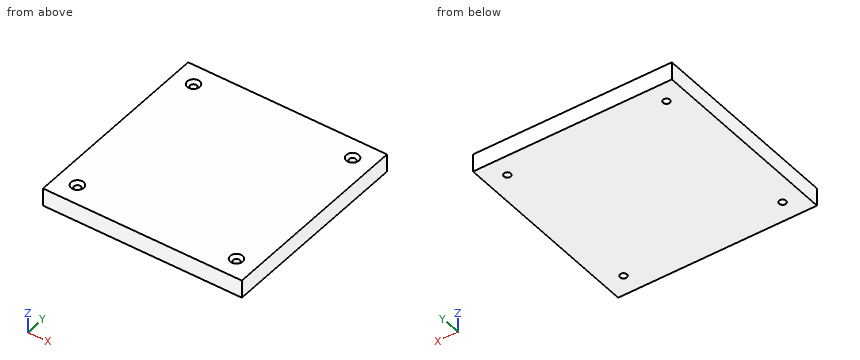
from build123d import *

# Parameters (mm, degrees)
SKETCH_1_W                  = 100
SKETCH_1_H                  = 100
EXTRUDE_1_DEPTH             = 9
HOLE_WIZARD_M3_1_AT_2_COUNT = 2
HOLE_WIZARD_M3_1_AT_2_PITCH = 80
HOLE_WIZARD_M3_1_AT_3_COUNT = 2
HOLE_WIZARD_M3_1_AT_3_PITCH = 113.13708499
HOLE_WIZARD_M3_1_AT_4_COUNT = 2
HOLE_WIZARD_M3_1_AT_4_PITCH = 80


with BuildPart() as part:
    # 草圖1 → 填料-伸長1 (new body)
    with BuildSketch(Plane.XY):
        Rectangle(SKETCH_1_W, SKETCH_1_H)
    extrude(amount=EXTRUDE_1_DEPTH)

    # 草圖4 → M3 平頭機械螺釘的錐孔1 (revolve, cut)
    with BuildSketch(Plane(origin=(-40, 40, 9), x_dir=(0, -1, 0), z_dir=(1, 0, 0))):
        Polygon((0, 0), (0, 9), (1.725, 9), (1.7, 8.975), (1.7, 1.45), (3.15, 0), align=None)
    hole_wizard_m3_1 = revolve(axis=Axis((-40, 40, 15.35), (0, 0, -1)), mode=Mode.SUBTRACT)

    # M3 平頭機械螺釘的錐孔1 at 2: M3 平頭機械螺釘的錐孔1 ×2
    with Locations(*[(i * HOLE_WIZARD_M3_1_AT_2_PITCH, 0, 0) for i in range(1, HOLE_WIZARD_M3_1_AT_2_COUNT)]):
        add(hole_wizard_m3_1, mode=Mode.SUBTRACT)

    # M3 平頭機械螺釘的錐孔1 at 3: M3 平頭機械螺釘的錐孔1 ×2
    with Locations(*[Vector(0.7071067811865476, -0.7071067811865476, 0) * (i * HOLE_WIZARD_M3_1_AT_3_PITCH) for i in range(1, HOLE_WIZARD_M3_1_AT_3_COUNT)]):
        add(hole_wizard_m3_1, mode=Mode.SUBTRACT)

    # M3 平頭機械螺釘的錐孔1 at 4: M3 平頭機械螺釘的錐孔1 ×2
    with Locations(*[(0, -i * HOLE_WIZARD_M3_1_AT_4_PITCH, 0) for i in range(1, HOLE_WIZARD_M3_1_AT_4_COUNT)]):
        add(hole_wizard_m3_1, mode=Mode.SUBTRACT)


solid = part.part
The model under review builds one solid part; all positions refer to its coordinate system, in mm. Round coordinates to 2 decimals unless told otherwise and drop trailing zeros. Order: outer loops, then holes, each group sorted by start corner. A loop starts at its lowest first (then second) coordinate and runs counter-clockwise, first axis right, second up. Notation, with made-up numbers: (26, 2.25) -> (55, 2.25) arc R14 ccw to (55, 14.25) -> close; hole circle Ø5 at (46, 17.5). An arc over 180 degrees is marked (long way). Use CSV: the item, a comma, the result in double quotes. Start each with the question number.
(1) Insertion check: pin 1 (3 mm diameter, centred on x = 40, y = 40, fed in from -Z). The pin has a flat end and moves straight along its axis. Give the tip position at first contact, or say it passes through.
(2) Wall thickness on probe 1 along Y at (x, z) = (-40, 4.25); probe 2 along Y at (x, z) = (40.5, 3.5): over which ranges is each line inside the solid? List them lowest first. Write a range as from..to.
(3) Consider section A-A on x = -40. Write out the cut boundary in (y, z) (3 decimals), and give its area (3 significant figures).
Responses:
1,pin 1,"through"
2,probe 1,"-50..-41.7, -38.3..38.3, 41.7..50"
2,probe 2,"-50..-41.62, -38.38..38.38, 41.62..50"
3,outline,"(-50, 0) -> (-41.725, 0) -> (-41.7, 0.025) -> (-41.7, 7.55) -> (-43.15, 9) -> (-50, 9) -> close; (-38.3, 0.025) -> (-38.275, 0) -> (38.275, 0) -> (38.3, 0.025) -> (38.3, 7.55) -> (36.85, 9) -> (-36.85, 9) -> (-38.3, 7.55) -> close; (41.7, 0.025) -> (41.725, 0) -> (50, 0) -> (50, 9) -> (43.15, 9) -> (41.7, 7.55) -> close"
3,area,"835 mm²"
